```python
from build123d import *

# Parameters (mm, degrees)
CROQUIS1_W                   = 3
CROQUIS1_H                   = 4.7
SALIENTE_EXTRUIR1_DEPTH      = 13
SALIENTE_EXTRUIR2_DEPTH      = 3
CORTAR_EXTRUIR1_DEPTH        = 17.5747549
CORTAR_EXTRUIR1_DEPTH_BACK   = 17.5747549
CROQUIS2_R                   = 1
REDONDEO1_R                  = 0.5
TALADROAVANZADO1_OUTLINE_R   = 1.2
TALADROAVANZADO1_DEPTH       = 1
TALADROAVANZADO1_DRAFT       = -45
TALADROAVANZADO1_2_OUTLINE_R = 1.2
TALADROAVANZADO1_2_DEPTH     = 1
TALADROAVANZADO1_2_DRAFT     = -45
REDONDEO2_R                  = 1.5
CORTAR_EXTRUIR2_REACH        = 16.132
CROQUIS4_R                   = 1.2


# Read off the part's stored shape, not the designer's step: TaladroAvanzado1
with BuildPart() as part:
    # Croquis1 → Saliente-Extruir1 (new body)
    with BuildSketch(Plane(origin=(0, 0, 0), x_dir=(1, 0, 0), z_dir=(0, 1, 0))):
        with Locations((-1.5, 0)):
            Rectangle(CROQUIS1_W, CROQUIS1_H)
        with Locations((1.5, 0)):
            Rectangle(CROQUIS1_W, CROQUIS1_H)
    extrude(amount=SALIENTE_EXTRUIR1_DEPTH)

    # Croquis1<3> → Saliente-Extruir2 (add)
    with BuildSketch(Plane(origin=(0, 0, 0), x_dir=(1, 0, 0), z_dir=(0, 1, 0))):
        with BuildLine():
            Line((3, 2.35), (3, 5.35))
            ThreePointArc((3, 5.35), (0, 8.35), (-3, 5.35))
            Line((-3, 5.35), (-3, 2.35))
            Line((-3, 2.35), (3, 2.35))
        make_face()
        with BuildLine():
            Line((3, -5.35), (3, -2.35))
            Line((3, -2.35), (-3, -2.35))
            Line((-3, -2.35), (-3, -5.35))
            ThreePointArc((-3, -5.35), (0, -8.35), (3, -5.35))
        make_face()
    extrude(amount=SALIENTE_EXTRUIR2_DEPTH)

    # Croquis2 → Cortar-Extruir1 (cut, two sides: drawn at the far end of the back side and taken through both)
    with BuildSketch(Plane(origin=(3, 0, 0), x_dir=(0, 0, -1), z_dir=(1, 0, 0)).offset(-CORTAR_EXTRUIR1_DEPTH_BACK)):
        with Locations((0, 10)):
            Circle(CROQUIS2_R)
    extrude(amount=CORTAR_EXTRUIR1_DEPTH + CORTAR_EXTRUIR1_DEPTH_BACK, mode=Mode.SUBTRACT)

    # Redondeo1
    redondeo1_edges = [part.edges().sort_by_distance(p)[0] for p in [
        (0, 3, 2.35),
        (0, 3, -2.35),
    ]]
    fillet(redondeo1_edges, radius=REDONDEO1_R)


with BuildPart() as taladroavanzado1_tool:
    # TaladroAvanzado1 outline → TaladroAvanzado1 (with draft: the straight prism first)
    with BuildSketch(Plane(origin=(0, 2, 0), x_dir=(1, 0, 0), z_dir=(0, 1, 0))):
        with Locations((0, 5.35)):
            Circle(TALADROAVANZADO1_OUTLINE_R)
    extrude(amount=TALADROAVANZADO1_DEPTH)
    # TaladroAvanzado1: the draft: its side faces are tilted about the plane it starts from
    taladroavanzado1_sides = [taladroavanzado1_tool.faces().sort_by_distance(p)[0] for p in [
        (-1.2, 2.5, -5.35),
    ]]
    draft(taladroavanzado1_sides, Plane(origin=(0, 2, 0), x_dir=(1, 0, 0), z_dir=(0, 1, 0)), TALADROAVANZADO1_DRAFT)


with BuildPart() as part_1:
    add(part.part)

    # TaladroAvanzado1: cut by taladroavanzado1_tool
    add(taladroavanzado1_tool.part, mode=Mode.SUBTRACT)


with BuildPart() as taladroavanzado1_2_tool:
    # TaladroAvanzado1 2 outline → TaladroAvanzado1 2 (with draft: the straight prism first)
    with BuildSketch(Plane(origin=(0, 2, 0), x_dir=(1, 0, 0), z_dir=(0, 1, 0))):
        with Locations((0, -5.35)):
            Circle(TALADROAVANZADO1_2_OUTLINE_R)
    extrude(amount=TALADROAVANZADO1_2_DEPTH)
    # TaladroAvanzado1 2: the draft: its side faces are tilted about the plane it starts from
    taladroavanzado1_2_sides = [taladroavanzado1_2_tool.faces().sort_by_distance(p)[0] for p in [
        (-1.2, 2.5, 5.35),
    ]]
    draft(taladroavanzado1_2_sides, Plane(origin=(0, 2, 0), x_dir=(1, 0, 0), z_dir=(0, 1, 0)), TALADROAVANZADO1_2_DRAFT)


with BuildPart() as part_2:
    add(part_1.part)

    # TaladroAvanzado1 2: cut by taladroavanzado1_2_tool
    add(taladroavanzado1_2_tool.part, mode=Mode.SUBTRACT)

    # Redondeo2
    redondeo2_edges = [part_2.edges().sort_by_distance(p)[0] for p in [
        (0, 13, -2.35),
        (0, 13, 2.35),
    ]]
    fillet(redondeo2_edges, radius=REDONDEO2_R)

    # Croquis4 → Cortar-Extruir2 (cut, up to next)
    with BuildSketch(Plane(origin=(0, 2, 0), x_dir=(1, 0, 0), z_dir=(0, 1, 0)), mode=Mode.PRIVATE) as cortar_extruir2_sk1:
        with Locations(Location((0, -5.35, 0), (0, 0, 270))):
            Circle(CROQUIS4_R)
    cortar_extruir2_tool1 = extrude(cortar_extruir2_sk1.sketch, amount=-CORTAR_EXTRUIR2_REACH, mode=Mode.PRIVATE) & part_2.part
    # Croquis4 → Cortar-Extruir2 (cut, up to next)
    with BuildSketch(Plane(origin=(0, 2, 0), x_dir=(1, 0, 0), z_dir=(0, 1, 0)), mode=Mode.PRIVATE) as cortar_extruir2_sk2:
        with Locations(Location((0, 5.35, 0), (0, 0, 270))):
            Circle(CROQUIS4_R)
    cortar_extruir2_tool2 = extrude(cortar_extruir2_sk2.sketch, amount=-CORTAR_EXTRUIR2_REACH, mode=Mode.PRIVATE) & part_2.part
    add(cortar_extruir2_tool1.solids().sort_by_distance((0, 2, 5.35))[0], mode=Mode.SUBTRACT)
    add(cortar_extruir2_tool2.solids().sort_by_distance((0, 2, -5.35))[0], mode=Mode.SUBTRACT)


solid = part_2.part
```
For this review, take the finished solid that the model builds, in its own axes (mm). A direction names the side the tool comes from. Round coordinates to 2 decimals unless told otherwise and drop trailing zeros. Order: outer loops, then holes, each group sorted by start corner. A loop starts at its lowest first (then second) coordinate and runs counter-clockwise, first axis right, second up. Notation, with made-up numbers: (25, -35.5) -> (67, -35.5) arc R30 ccw to (67, -6.5) -> close; hole circle Ø3 at (-24.5, 11). An arc over 180 degrees is marked (long way). Use a Markdown table: item, result.
Item 1: Take a section at C-C (x = -2.4). State the section outline as (y, z) points.
Resolved:
| item | result |
|---|---|
| outline | (0, -7.15) -> (3, -7.15) -> (3, -2.85) arc R0.5 cw to (3.5, -2.35) -> (11.5, -2.35) arc R1.5 ccw to (13, -0.85) -> (13, 0.85) arc R1.5 ccw to (11.5, 2.35) -> (3.5, 2.35) arc R0.5 cw to (3, 2.85) -> (3, 7.15) -> (0, 7.15) -> close; hole circle Ø2 at (10, 0) |
Item 2: For pin 1 (1.6 mm diameter, centred on x = 0, z = 6, fed in from +Y); pin 2 (1.8 mm diameter, centred on x = 1.5, y = 6, fed in from -Z); pin 3 (2.5 mm diameter, centred on y = 10, z = 0, fed in from -X); pin 4 (3 mm diameter, centred on x = 0.5, y = 8, fed in from +Z), all flat-tipped, find the tip position at first contact; note any pin that passes through.
Resolved:
| item | result |
|---|---|
| pin 1 | stops at y = 2.25 |
| pin 2 | stops at z = -2.35 |
| pin 3 | stops at x = -3 |
| pin 4 | stops at z = 2.35 |
Item 3: Machinability: for faces 5 (the cylindrical face through (0.07, 1.48, -8.35)), 6 (the flat face through (-2, 3, -4)), 7 (the flat face through (0, 7, 2.35)), which of the approach directions +Z, -Z, +X, -X, +Y, -Y give a long, thin tool a straight path to every point of the face, cutting with its end or side? Answer none if there is none.
Resolved:
| item | result |
|---|---|
| face 5 | -Z, +Y, -Y |
| face 6 | -Z, +X, -X, +Y |
| face 7 | +Z, +X, -X, +Y |
Item 4: Take a section at A-A (x = 0). State the section outline as (y, z) points.
Resolved:
| item | result |
|---|---|
| outline | (0, -8.35) -> (3, -8.35) -> (3, -7.55) -> (2, -6.55) -> (0, -6.55) -> close; (0, -4.15) -> (2, -4.15) -> (3, -3.15) -> (3, -2.85) arc R0.5 cw to (3.5, -2.35) -> (11.5, -2.35) arc R1.5 ccw to (13, -0.85) -> (13, 0.85) arc R1.5 ccw to (11.5, 2.35) -> (3.5, 2.35) arc R0.5 cw to (3, 2.85) -> (3, 3.15) -> (2, 4.15) -> (0, 4.15) -> close; (0, 6.55) -> (2, 6.55) -> (3, 7.55) -> (3, 8.35) -> (0, 8.35) -> close; hole circle Ø2 at (10, 0) |
Item 5: For line 1 along Z through (x, y) = (0, 1.15); line 2 along Y through (x, z) = (0.4, 0); line 3 along Z through (x, y) = (1.7, 10), list the stretches that pass through material, from the lowest coordinate up. Write a range as [from, to].
Resolved:
| item | result |
|---|---|
| line 1 | z = [-8.35, -6.55], [-4.15, 4.15], [6.55, 8.35] |
| line 2 | y = [0, 9], [11, 13] |
| line 3 | z = [-2.35, -1], [1, 2.35] |
Item 6: Draft analysis for pull direction Y (two halves, no side actions). For faces 1 (the cylindrical face through (0, 11, 0)), 2 (the flat face through (0, 7, -2.35)), 3 (the flat face through (0, 0, 0)), 4 (the flat face through (0, 13, 0)), state which applies: +Y half, -Y half, draft (parallel to the pull), parting line (faces both ways), or undercut.
Resolved:
| item | result |
|---|---|
| face 1 | undercut |
| face 2 | draft |
| face 3 | -Y half |
| face 4 | +Y half |
Item 7: Take a section at D-D (z = 0). State the section outline as (x, y) points, plus the area to 3 significant figures.
Resolved:
| item | result |
|---|---|
| outline | (-3, 0) -> (3, 0) -> (3, 9) -> (-3, 9) -> close; (-3, 11) -> (3, 11) -> (3, 13) -> (-3, 13) -> close |
| area | 66.0 mm² |
Item 8: Take a section at B-B (y = 10). State the section outline as (x, z) points.
Resolved:
| item | result |
|---|---|
| outline | (-3, -2.35) -> (3, -2.35) -> (3, -1) -> (-3, -1) -> close; (-3, 1) -> (3, 1) -> (3, 2.35) -> (-3, 2.35) -> close |
